Model file for the job. Use its own axes, mm. A direction names the side the tool comes from. Coordinates: 2 decimals unless noted, no trailing zeros. Order: outer loops, then holes, each group sorted by start corner. A loop starts at its lowest first (then second) coordinate and runs counter-clockwise, first axis right, second up. Notation, with made-up numbers: (48, 19) -> (88, 19) arc R19 ccw to (88, 38) -> close; hole circle Ø3 at (86, -23). An arc over 180 degrees is marked (long way). Return JSON: item names as keys, results as strings. Group by question number.
1) Probe line 1 (Z direction, x = 31, y = 9.75); line 2 (Z direction, x = 27, y = 3.5); line 3 (Y direction, x = 70, z = 87). List the from-to ranges inside material, lowest first.
2) Cut at C-C (z = 54). Write the cut outline in (x, y).
3) Cut at D-D (x = 94). Write the cut outline in (y, z), and give its area (3 significant figures).
4) Pull direction Z, two halves, no side cores. Call faces 1 (the flat face through (0, 13, 47)), 2 (the flat face through (56, 9, 83.75)): +Z half, -Z half, draft (parallel to the pull), parting line (faces both ways), or undercut.
5) Flat gauge pins, fed straight in: pin 1 (12.5 mm diameter, centred on y = 14, z = 51.5, fed in from +X); pin 2 (4 mm diameter, centred on x = 86.5, y = 6.5, fed in from -Z); pin 3 (13.5 mm diameter, centred on x = 120, z = 83.5, fed in from +Y); pin 4 (0.9 mm diameter, centred on y = -2, z = 4.5, fed in from -X). Where does each tip first touch, or does it go through?
6) Cut at B-B (y = 11). Write the cut outline in (x, z), and give its area (3 significant figures).
7) Which spindle directions (+Z, -Z, +X, -X, +Y, -Y) get a long thin tool onto all of the face, cutting with end or side? Do faces 3 (the flat face through (105, 10, 48)), 4 (the cylindrical face through (52.35, 18.29, 11.05)), 5 (the flat face through (3, 6.5, 49)). Say none if no direction does.
8) Cut at A-A (x = 124.5). Write the cut outline in (y, z).
from build123d import *

# Parameters (mm, degrees)
SKETCH1_W                = 105
SKETCH1_H                = 25
BOSS_EXTRUDE4_DEPTH      = 19
BOSS_EXTRUDE5_DEPTH      = 5.5
BOSS_EXTRUDE5_DEPTH_BACK = 24
SKETCH4_W                = 105
SKETCH4_H                = 12.5
FILLET3_R                = 2.5
BOSS_EXTRUDE7_DEPTH      = 2.5
BOSS_EXTRUDE7_DEPTH_BACK = 22
SKETCH7_W                = 6.5
SKETCH7_H                = 11.5
CUT_EXTRUDE1_DEPTH       = 96


with BuildPart() as part:
    # Sketch1 → Boss-Extrude4 (new body)
    # profile 1 of 5: a face of its own
    with BuildSketch(Plane(origin=(0, 0, 0), x_dir=(1, 0, 0), z_dir=(0, 1, 0))):
        Polygon((136, 0), (94, 0), (94, -17), (129, -17), (136, -10), align=None)
    # profile 2 of 5: a face of its own
    with BuildSketch(Plane(origin=(0, 0, 0), x_dir=(1, 0, 0), z_dir=(0, 1, 0))):
        Polygon((94, 0), (0, 0), (0, -35.5), (105, -35.5), (110.5, -35.5), (129, -17), (94, -17), align=None)
        with BuildLine():
            ThreePointArc((26.584181208, -22.999838941), (21.042251663, -17.542090604), (26.5, -12.000161059))
            Line((26.5, -12.000161059), (77.5, -11.609854936))
            ThreePointArc((77.5, -11.609854936), (83.041929546, -17.067603273), (77.584181208, -22.609532819))
            Line((77.584181208, -22.609532819), (26.584181208, -22.999838941))
        make_face(mode=Mode.SUBTRACT)
    # profile 3 of 5: a face of its own
    with BuildSketch(Plane(origin=(0, 0, 0), x_dir=(1, 0, 0), z_dir=(0, 1, 0))):
        with Locations((52.5, -48)):
            Rectangle(SKETCH1_W, SKETCH1_H)
    # profile 4 of 5: a face of its own
    with BuildSketch(Plane(origin=(0, 0, 0), x_dir=(1, 0, 0), z_dir=(0, 1, 0))):
        Polygon((105, -60.5), (0, -60.5), (0, -96), (94, -96), (94, -79), (129, -79), (110.5, -60.5), align=None)
        with BuildLine():
            ThreePointArc((30.542090604, -83.75), (25.042090604, -78.25), (30.542090604, -72.75))
            Line((30.542090604, -72.75), (81.542090604, -72.75))
            ThreePointArc((81.542090604, -72.75), (87.042090604, -78.25), (81.542090604, -83.75))
            Line((81.542090604, -83.75), (30.542090604, -83.75))
        make_face(mode=Mode.SUBTRACT)
    # profile 5 of 5: a face of its own
    with BuildSketch(Plane(origin=(0, 0, 0), x_dir=(1, 0, 0), z_dir=(0, 1, 0))):
        Polygon((94, -79), (94, -96), (136, -96), (136, -86), (129, -79), align=None)
    extrude(amount=BOSS_EXTRUDE4_DEPTH)

    # Sketch4 → Boss-Extrude5 (add, two sides: drawn at the far end of the back side and taken through both)
    with BuildSketch(Plane(origin=(0, 19, 0), x_dir=(1, 0, 0), z_dir=(0, 1, 0)).offset(-BOSS_EXTRUDE5_DEPTH_BACK)):
        with Locations((52.5, -41.75)):
            Rectangle(SKETCH4_W, SKETCH4_H)
        with Locations((52.5, -54.25)):
            Rectangle(SKETCH4_W, SKETCH4_H)
    extrude(amount=BOSS_EXTRUDE5_DEPTH + BOSS_EXTRUDE5_DEPTH_BACK)

    # Fillet3
    fillet3_edges = [part.edges().sort_by_distance(p)[0] for p in [
        (56.042090604, 19, 72.75),
        (56.042090604, 0, 72.75),
        (25.042090604, 0, 78.25),
        (56.042090604, 0, 83.75),
        (87.042090604, 0, 78.25),
        (52, 0, 11.805007997),
        (21.042251663, 0, 17.542090604),
        (52.084181208, 0, 22.80468588),
        (83.041929546, 0, 17.067603273),
        (83.041929546, 19, 17.067603273),
        (52.084181208, 19, 22.80468588),
        (21.042251663, 19, 17.542090604),
        (52, 19, 11.805007997),
        (87.042090604, 19, 78.25),
        (56.042090604, 19, 83.75),
        (25.042090604, 19, 78.25),
    ]]
    fillet(fillet3_edges, radius=FILLET3_R)

    # Sketch5 → Boss-Extrude7 (add, two sides: drawn at the far end of the back side and taken through both)
    with BuildSketch(Plane(origin=(0, 19, 0), x_dir=(1, 0, 0), z_dir=(0, 1, 0)).offset(-BOSS_EXTRUDE7_DEPTH_BACK)):
        Polygon((101, 0), (101, -17), (129, -17), (136, -10), (136, 0), align=None)
        Polygon((136, -86), (129, -79), (101, -79), (101, -96), (136, -96), align=None)
    extrude(amount=BOSS_EXTRUDE7_DEPTH + BOSS_EXTRUDE7_DEPTH_BACK)

    # Sketch7 → Cut-Extrude1 (cut)
    with BuildSketch(Plane.XY.offset(96)):
        with Locations((3.25, 0.75)):
            Rectangle(SKETCH7_W, SKETCH7_H)
    extrude(amount=-CUT_EXTRUDE1_DEPTH, mode=Mode.SUBTRACT)


solid = part.part
Answers below:
{
 "1": {"line 1": "z = 0 to 11.97, 22.97 to 72.75, 83.75 to 96", "line 2": "z = 0 to 12, 23 to 74.04, 82.46 to 96", "line 3": "y = 0 to 19"},
 "2": {"outline": "(0, 6.5) -> (6.5, 6.5) -> (6.5, -5) -> (105, -5) -> (105, 24.5) -> (0, 24.5) -> close"},
 "3": {"outline": "(-5, 35.5) -> (0, 35.5) -> (0, 0) -> (19, 0) -> (19, 35.5) -> (24.5, 35.5) -> (24.5, 60.5) -> (19, 60.5) -> (19, 96) -> (0, 96) -> (0, 60.5) -> (-5, 60.5) -> close", "area": "2,090 mm^2"},
 "4": {"face 1": "draft", "face 2": "undercut"},
 "5": {"pin 1": "stops at x = 105", "pin 2": "stops at z = 0", "pin 3": "stops at y = 21.5", "pin 4": "stops at x = 101"},
 "6": {"outline": "(0, 0) -> (136, 0) -> (136, 10) -> (110.5, 35.5) -> (105, 35.5) -> (105, 60.5) -> (110.5, 60.5) -> (136, 86) -> (136, 96) -> (0, 96) -> close; hole (26.5, 12) -> (77.5, 11.61) arc R5.5 ccw to (77.58, 22.61) -> (26.58, 23) arc R5.5 ccw to start; hole (30.54, 72.75) -> (81.54, 72.75) arc R5.5 ccw to (81.54, 83.75) -> (30.54, 83.75) arc R5.5 ccw to start", "area": "10,300 mm^2"},
 "7": {"face 3": "+X, +Y, -Y", "face 4": "+Y", "face 5": "+Z, -Z, -X, -Y"},
 "8": {"outline": "(-3, 0) -> (21.5, 0) -> (21.5, 17) -> (19, 17) -> (19, 21.5) -> (0, 21.5) -> (0, 17) -> (-3, 17) -> close; (-3, 79) -> (0, 79) -> (0, 74.5) -> (19, 74.5) -> (19, 79) -> (21.5, 79) -> (21.5, 96) -> (-3, 96) -> close"}
}
